```python
from build123d import *

# Parameters (mm, degrees)
F0_W     = 0.82
F0_H     = 0.8
F1_DEPTH = 2
F2_DEPTH = 0.8


with BuildPart() as f1:
    # F0 (on Top) → F1 (new body)
    with BuildSketch(Plane.XY):
        Polygon((-10.41, 0.41), (-0.41, 0.41), (-0.41, 10.41), (0.41, 10.41), (0.41, 0.41), (10.41, 0.41), (10.41, -0.41), (0.41, -0.41), (0.41, -1.21), (1.21, -1.21), (11.21, -1.21), (11.21, 1.21), (1.21, 1.21), (1.21, 11.21), (-1.21, 11.21), (-1.21, 1.21), (-11.21, 1.21), (-11.21, -1.21), (-1.21, -1.21), (-0.41, -1.21), (-0.41, -0.41), (-10.41, -0.41), align=None)
        with Locations((0, -0.81)):
            Rectangle(F0_W, F0_H)
    extrude(amount=F1_DEPTH)

    # F0 (on Top) + F1_face (on face) → F2 (join)
    with BuildSketch(Plane.XY):
        Polygon((-1.21, 11.21), (-11.21, 1.21), (-1.21, 1.21), align=None)
        Polygon((1.21, 1.21), (11.21, 1.21), (1.21, 11.21), align=None)
        Polygon((-10.41, 0.41), (-0.41, 0.41), (-0.41, 10.41), (0.41, 10.41), (0.41, 0.41), (10.41, 0.41), (10.41, -0.41), (0.41, -0.41), (0.41, -1.21), (1.21, -1.21), (11.21, -1.21), (11.21, 1.21), (1.21, 1.21), (1.21, 11.21), (-1.21, 11.21), (-1.21, 1.21), (-11.21, 1.21), (-11.21, -1.21), (-1.21, -1.21), (-0.41, -1.21), (-0.41, -0.41), (-10.41, -0.41), align=None)
        Polygon((-0.41, 10.41), (-0.41, 0.41), (-10.41, 0.41), (-10.41, -0.41), (-0.41, -0.41), (0.41, -0.41), (10.41, -0.41), (10.41, 0.41), (0.41, 0.41), (0.41, 10.41), align=None)
        with Locations((0, -0.81)):
            Rectangle(F0_W, F0_H)
    with BuildSketch(Plane(origin=(0, 1.991576, 2), x_dir=(1, 0, 0), z_dir=(0, 0, 1))):
        Polygon((11.21, -3.201576), (11.21, -0.781576), (1.21, -0.781576), (1.21, 9.218424), (-1.21, 9.218424), (-1.21, -0.781576), (-11.21, -0.781576), (-11.21, -3.201576), align=None)
        Polygon((-10.41, -2.401576), (-10.41, -1.581576), (-0.41, -1.581576), (-0.41, 8.418424), (0.41, 8.418424), (0.41, -1.581576), (10.41, -1.581576), (10.41, -2.401576), align=None, mode=Mode.SUBTRACT)
    extrude(amount=-F2_DEPTH)


solid = f1.part
```
Work out the finished part from the listing and answer in its coordinate system (mm). A direction names the side the tool comes from. Coordinates: 2 decimals unless noted, no trailing zeros. Write each loop counter-clockwise with the first axis right and the second up, starting at its lowest first coordinate (ties: lowest second). Pieces come first, ordered by that corner, then holes. Notation, with made-up numbers: (-32, 6) - (-17, 6) arc R21 ccw to (-17, 24) - close; hole circle Ø8 at (5, -15). An arc over 180 degrees is marked (long way). Answer as a JSON object with one key per item and string values.
Q1. For a pull along Y with two mould halves and no side action, classify faces 1 (the flat face through (0, 10.41, 1)), 2 (the flat face through (10.41, 0, 1)), 3 (the flat face through (6, 1.21, 1)), 4 (the flat face through (-4, 4, 0)) as pulls with the +Y half, pulls with the -Y half, needs draft (parallel to the pull), parting line crosses it, or undercut.
Results list:
{"face 1": "undercut", "face 2": "undercut", "face 3": "pulls with the +Y half", "face 4": "needs draft"}
Q2. Given pin 1 Ø1.6 at (x, z) = (-7, 1.5) entering from +Y; pin 2 Ø0.6 at (y, z) = (4.5, 0.5) entering from -X; pin 3 Ø1.5 at (y, z) = (3.5, 0.5) entering from -X, each flat-ended and moving along its own axis, determine where each tip first touches the part or whether it passes through.
Results list:
{"pin 1": "stops at y = 1.21", "pin 2": "stops at x = -1.21", "pin 3": "stops at x = -9.48"}
Q3. Find section B-B (y = 9). Write down the section's boundary in (x, z), plus the area to 3 significant figures.
Results list:
{"outline": "(-3.42, -0.8) - (3.42, -0.8) - (3.42, 0) - (1.21, 0) - (1.21, 2) - (0.41, 2) - (0.41, 0) - (-0.41, 0) - (-0.41, 2) - (-1.21, 2) - (-1.21, 0) - (-3.42, 0) - close", "area": "8.67 mm^2"}
Q4. Find section C-C (x = -6). Write down the section's boundary in (y, z).
Results list:
{"outline": "(-1.21, -0.8) - (6.42, -0.8) - (6.42, 0) - (1.21, 0) - (1.21, 2) - (0.41, 2) - (0.41, 0) - (-0.41, 0) - (-0.41, 2) - (-1.21, 2) - close"}
Q5. Find section A-A (z = 1.4). Write down the section's boundary in (x, y).
Results list:
{"outline": "(-11.21, -1.21) - (11.21, -1.21) - (11.21, 1.21) - (1.21, 1.21) - (1.21, 11.21) - (-1.21, 11.21) - (-1.21, 1.21) - (-11.21, 1.21) - close; hole (-10.41, -0.41) - (10.41, -0.41) - (10.41, 0.41) - (0.41, 0.41) - (0.41, 10.41) - (-0.41, 10.41) - (-0.41, 0.41) - (-10.41, 0.41) - close"}
Q6. Consider L1, parallel to Y at x = -5.75, z = 1.75; L2, parallel to Y at x = -1, z = 0.5. Determine where each line is inside the solid, lowest interval first. Write a range as from..to.
Results list:
{"L1": "y = -1.21..-0.41, 0.41..1.21", "L2": "y = -1.21..-0.41, 0.41..11.21"}
Q7. Which of the six approach directions +Z, -Z, +X, -X, +Y, -Y give full straight-line access (tool end or side, diameter ignored) to faces 5 (the flat face through (11.21, 0, 1)), 6 (the flat face through (-1.21, 6, 1)), 7 (the flat face through (4, 4, 0)), 8 (the flat face through (-0.41, 5, 1)), 9 (the flat face through (-11.21, 0, 1))?
Results list:
{"face 5": "+Z, -Z, +X, +Y, -Y", "face 6": "+Z, -X, +Y", "face 7": "+Z, +X, +Y", "face 8": "+Z", "face 9": "+Z, -Z, -X, +Y, -Y"}
Q8. Find section D-D (z = -0.5). Write down the section's boundary in (x, y), plus the area to 3 significant figures.
Results list:
{"outline": "(-11.21, -1.21) - (11.21, -1.21) - (11.21, 1.21) - (1.21, 11.21) - (-1.21, 11.21) - (-11.21, 1.21) - close", "area": "178 mm^2"}
